```python
from build123d import *

# Parameters (mm, degrees)
BOSS_EXTRUDE1_DEPTH        = 6
M5_CLEARANCE_HOLE1_D       = 5.3
M3_CLEARANCE_HOLE1_D       = 3.2
F_22_0_22_DIAMETER_HOLE1_D = 22
FILLET1_R                  = 1


with BuildPart() as part:
    # Sketch1 → Boss-Extrude1 (new body)
    with BuildSketch(Plane(origin=(0, 0, 0), x_dir=(1, 0, 0), z_dir=(0, 1, 0))):
        Polygon((0, 0), (81, 0), (81, 42), (42, 42), (42, 81), (0, 81), align=None)
    extrude(amount=BOSS_EXTRUDE1_DEPTH)

    # M5 Clearance Hole1 (through all)
    with Locations(Plane(origin=(0, 6, 0), x_dir=(1, 0, 0), z_dir=(0, 1, 0))):
        with Locations((10, 30), (30, 30), (30, 10), (10, 10)):
            Hole(M5_CLEARANCE_HOLE1_D / 2)

    # M3 Clearance Hole1 (through all)
    with Locations(Plane(origin=(0, 6, 0), x_dir=(1, 0, 0), z_dir=(0, 1, 0))):
        with Locations((5.5, 44.5), (36.5, 44.5), (36.5, 75.5), (5.5, 75.5), (44.5, 36.5), (44.5, 5.5), (75.5, 5.5), (75.5, 36.5)):
            Hole(M3_CLEARANCE_HOLE1_D / 2)

    # Ø22.0 (22) Diameter Hole1 (through all)
    with Locations(Plane(origin=(0, 6, 0), x_dir=(1, 0, 0), z_dir=(0, 1, 0))):
        with Locations((60, 21), (21, 60)):
            Hole(F_22_0_22_DIAMETER_HOLE1_D / 2)

    # Fillet1
    fillet1_edges = [part.edges().sort_by_distance(p)[0] for p in [
        (0, 3, -81),
        (42, 3, -81),
        (81, 3, -42),
        (81, 3, 0),
        (0, 3, 0),
    ]]
    fillet(fillet1_edges, radius=FILLET1_R)


solid = part.part
```
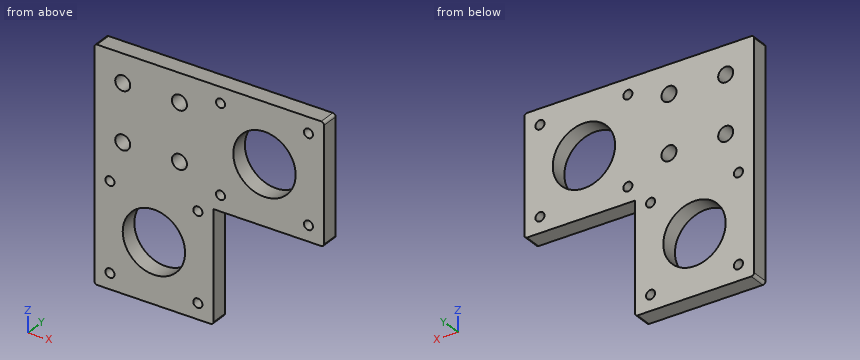
Read the model definition and answer for the solid it produces. Units are mm, in the model's axes. Coordinates: 2 decimals unless noted, no trailing zeros. Write each loop counter-clockwise with the first axis right and the second up, starting at its lowest first coordinate (ties: lowest second). Pieces come first, ordered by that corner, then holes. Notation, with made-up numbers: (-12, 14) -> (26, 14) arc R25 ccw to (26, 30) -> close; hole circle Ø1 at (70.5, 66.5). An arc over 180 degrees is marked (long way). Return JSON: item names as keys, results as strings.
1. A cutting plane is placed at C-C (x = 36.5). Determine the outline of the cut face in (y, z).
Found:
{"outline": "(0, -81) -> (6, -81) -> (6, -77.1) -> (0, -77.1) -> close; (0, -73.9) -> (6, -73.9) -> (6, -46.1) -> (0, -46.1) -> close; (0, -42.9) -> (6, -42.9) -> (6, 0) -> (0, 0) -> close"}
2. A cutting plane is placed at D-D (z = -44.5). Determine the outline of the cut face in (x, y), and give its area (3 significant figures).
Found:
{"outline": "(0, 0) -> (3.9, 0) -> (3.9, 6) -> (0, 6) -> close; (7.1, 0) -> (34.9, 0) -> (34.9, 6) -> (7.1, 6) -> close; (38.1, 0) -> (42, 0) -> (42, 6) -> (38.1, 6) -> close", "area": "214 mm2"}
3. Find the intervals of material crossed by line 1 along Z through (x, y) = (5.5, 1.3); line 2 along X through (y, z) = (2.5, -75.5); line 3 along X through (y, z) = (4.1, -5.5), in increasing order. Write a range as from..to.
Found:
{"line 1": "-81..-77.1, -73.9..-46.1, -42.9..0", "line 2": "0..3.9, 7.1..34.9, 38.1..42", "line 3": "0..42.9, 46.1..73.9, 77.1..81"}
4. A cutting plane is placed at B-B (y = 4.4). Give the number of separate pieces and of enclosed holes in the cut face, and give its area (3 significant figures).
Found:
{"separate pieces": "1", "enclosed holes": "14", "area": "4,130 mm2"}
5. Each of these flat-tipped pins is pushed along its axis until it touches: P1, Ø1.9, axis at x = 36.5, z = -44.5, coming from the +Y side; P2, Ø2, axis at x = 52.5, y = 2, coming from the -Z side. Where does it stop, or does it pass through?
Found:
{"P1": "through", "P2": "z = -42"}
6. A cutting plane is placed at A-A (z = -21). Determine the outline of the cut face in (x, y), and give its area (3 significant figures).
Found:
{"outline": "(0, 0) -> (49, 0) -> (49, 6) -> (0, 6) -> close; (71, 0) -> (81, 0) -> (81, 6) -> (71, 6) -> close", "area": "354 mm2"}
